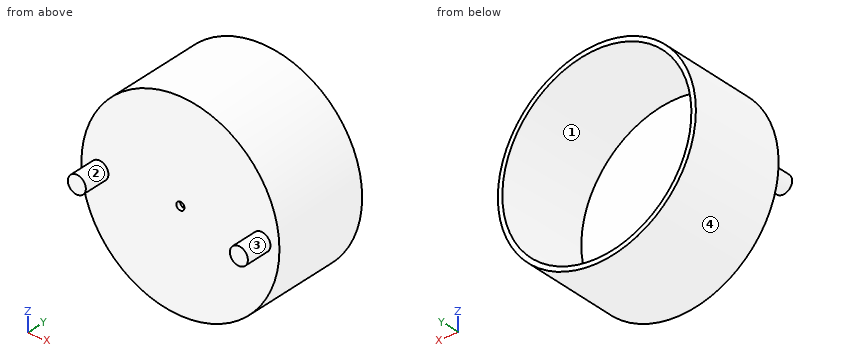
```python
from build123d import *

# Parameters (mm, degrees)
CUT_EXTRUDE2_REACH  = 192.526
MOTOR_HOLE_R        = 4.5
STABLIZING_POLES_R  = 10
BOSS_EXTRUDE1_DEPTH = 30


with BuildPart() as part:
    # Compartment → Revolve1 (revolve)
    with BuildSketch(Plane.XY, mode=Mode.PRIVATE) as revolve1_sk:
        Polygon((110, -80), (0, -80), (0, -75), (105, -75), (105, 30), (110, 30), align=None)
    revolve(revolve1_sk.sketch.rotate(Axis((0, 0, 0), (0, 1, 0)), 90), axis=Axis((0, 0, 0), (0, 1, 0)))

    # Motor Hole → Cut-Extrude2 (cut, up to next)
    with BuildSketch(Plane.XZ.offset(80), mode=Mode.PRIVATE) as cut_extrude2_sk1:
        with Locations(Location((0, 0, 0), (0, 0, 270))):
            Circle(MOTOR_HOLE_R)
    cut_extrude2_tool1 = extrude(cut_extrude2_sk1.sketch, amount=-CUT_EXTRUDE2_REACH, mode=Mode.PRIVATE) & part.part
    add(cut_extrude2_tool1.solids().sort_by_distance((0, -80, 0))[0], mode=Mode.SUBTRACT)

    # Stablizing poles → Boss-Extrude1 (add)
    with BuildSketch(Plane.XZ.offset(80)):
        with Locations(Location((-90, 0, 0), (0, 0, 270))):
            Circle(STABLIZING_POLES_R)
        with Locations(Location((90, 0, 0), (0, 0, 270))):
            Circle(STABLIZING_POLES_R)
    extrude(amount=BOSS_EXTRUDE1_DEPTH)


solid = part.part
```
Read the model definition and answer for the solid it produces. Units are mm, in the model's axes. Face numbers are marked on the shaded views. A direction names the side the tool comes from. Give positions to 0.01 mm unless a question says otherwise; leave off trailing zeros. Write each loop counter-clockwise with the first axis right and the second up, starting at its lowest first coordinate (ties: lowest second). Pieces come first, ordered by that corner, then holes. Notation, with made-up numbers: (76.5, -6.75) - (126.5, -6.75) arc R29 cw to (126.5, 18.25) - close; hole circle Ø7 at (-12, -26). An arc over 180 degrees is marked (long way). Write item = value, one per line. Start each with the question number.
Item 1: Find section C-C (y = -97). Give the vertices of the cut face in (x, z), then the cut area to 3 significant figures.
Item 2: Each of these flat-tipped pins is pushed along its axis until it touches: P1, Ø10, axis at x = 61, z = 57, coming from the -Y side; P2, Ø5, axis at y = -1, z = 32.5, coming from the +X side; P3, Ø2, axis at y = -55, z = -85.5, coming from the -X side. Where does it stop, or does it pass through?
Item 3: The mould has two halves that part along X. Classify the marked faces 3 and 4: +X half, -X half, draft (parallel to the pull), parting line (faces both ways), or undercut.
Item 4: Find section A-A (x = 0). Give the vertices of the cut face in (y, z).
Item 5: Find the intervals of material crossed by probe 1 along Z at (x, y) = (-1, 22); probe 2 along X at (y, z) = (-77.45, 0); probe 3 along Y at (x, z) = (23.5, 60), in increasing order. Write a range as [from, to].
Item 6: Find section B-B (z = 0). Give the vertices of the cut face in (x, y).
Item 7: A tool of negligible diameter and unlimited length cuts with its end or side. For the marked faces 1 and 2, from which of +Z, -Z, +X, -X, +Y, -Y can it reach the whole face along a straight path? Write none if from no direction.
Item 8: Find section D-D (z = 66.5). Give the vertices of the cut face in (x, y).
Response:
q1.outline = circle Ø20 at (-90, 0); circle Ø20 at (90, 0)
q1.area = 628 mm²
q2.P1 = -80
q2.P2 = 105.83
q2.P3 = -70.43
q3.face_3 = undercut
q3.face_4 = parting line
q4.outline = (-80, -110) - (30, -110) - (30, -105) - (-75, -105) - (-75, -4.5) - (-80, -4.5) - close; (-80, 4.5) - (-75, 4.5) - (-75, 105) - (30, 105) - (30, 110) - (-80, 110) - close
q5.probe_1 = [-110, -105], [105, 110]
q5.probe_2 = [-110, -4.5], [4.5, 110]
q5.probe_3 = [-80, -75]
q6.outline = (-110, -80) - (-100, -80) - (-100, -110) - (-80, -110) - (-80, -80) - (-4.5, -80) - (-4.5, -75) - (-105, -75) - (-105, 30) - (-110, 30) - close; (4.5, -80) - (80, -80) - (80, -110) - (100, -110) - (100, -80) - (110, -80) - (110, 30) - (105, 30) - (105, -75) - (4.5, -75) - close
q7.face_1 = +Y
q7.face_2 = -Y
q8.outline = (-87.62, -80) - (87.62, -80) - (87.62, 30) - (81.26, 30) - (81.26, -75) - (-81.26, -75) - (-81.26, 30) - (-87.62, 30) - close
